Study the drawing (mm; zero at the part's minimum x, y, z) and answer. A direction names the side the tool comes from. Round coordinates to 2 decimals unless told otherwise and drop trailing zeros. Loops run counter-clockwise (first coordinate to the right, second up) from the corner with the lowest first, then second, coordinate; pieces in that order, holes last. Notation, with made-up numbers: (57.5, 70) - (95.5, 70) arc R26 ccw to (95.5, 95) - close; hole circle Ø11 at (12.25, 5.25). An arc over 180 degrees is marked (long way). One line per item, written item: value.
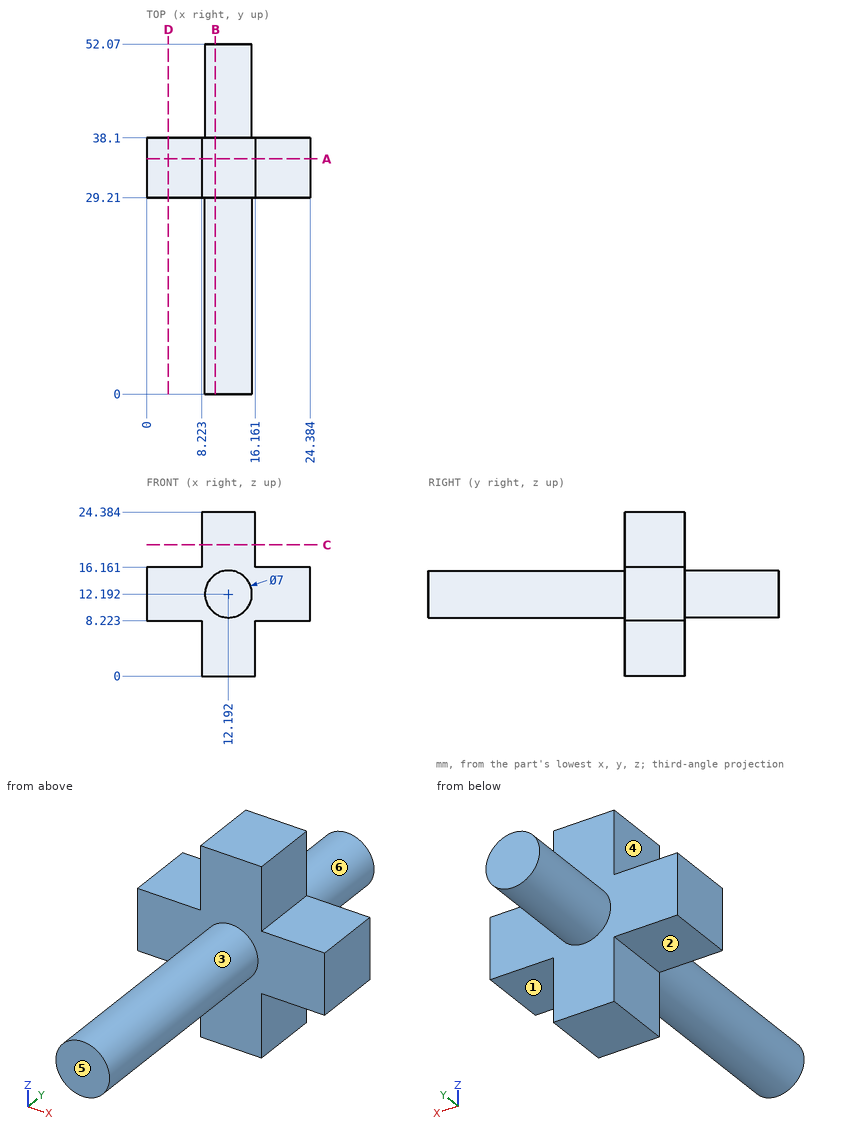
1) A cutting plane is placed at D-D on x = 3.25. Give the vertices of the cut face in (y, z).
Final values:
outline: (29.21, 8.22) - (38.1, 8.22) - (38.1, 16.16) - (29.21, 16.16) - close
2) For a pull along X with two mould halves and no side action, classify the marked faces 4, 5 and 6 as released by +X, released by -X, zero draft, split by the parting line, or undercut.
Final values:
face 4: released by -X
face 5: zero draft
face 6: split by the parting line
3) A cutting plane is placed at B-B on x = 10.25. Give the vertices of the cut face in (y, z).
Final values:
outline: (0, 9.28) - (29.21, 9.28) - (29.21, 0) - (38.1, 0) - (38.1, 9.28) - (52.07, 9.28) - (52.07, 15.1) - (38.1, 15.1) - (38.1, 24.38) - (29.21, 24.38) - (29.21, 15.1) - (0, 15.1) - close
4) For the marked faces 1, 2 and 3, determine the directions among +Z, -Z, +X, -X, +Y, -Y from which every point of the face is accessible in a straight line to the end or side of a thin tool.
Final values:
face 1: -Z, +X, +Y, -Y
face 2: -Z, -X, +Y, -Y
face 3: -Y
5) A cutting plane is placed at C-C on z = 19.5. Give the vertices of the cut face in (x, y).
Final values:
outline: (8.22, 29.21) - (16.16, 29.21) - (16.16, 38.1) - (8.22, 38.1) - close
6) Consider L1, parallel to Y at x = 23, z = 12.5; L2, parallel to Z at x = 3, y = 33; L3, parallel to Z at x = 13, y = 43.5. Determine where each line is inside the solid, lowest interval first.
Final values:
L1: 29.21 to 38.1
L2: 8.22 to 16.16
L3: 8.79 to 15.6
7) Each of these flat-tipped pins is pushed along its axis until it touches: pin 1 Ø2.5 at (x, y) = (22, 35) entering from +Z; pin 2 Ø4 at (y, z) = (35.5, 20) entering from -X; pin 3 Ø10 at (x, z) = (21, 15.5) entering from -Y. Where does it stop, or does it pass through?
Final values:
pin 1: z = 16.16
pin 2: x = 8.22
pin 3: y = 29.21
8) A cutting plane is placed at A-A on y = 35. Give the vertices of the cut face in (x, z), and give its area (3 significant figures).
Final values:
outline: (0, 8.22) - (8.22, 8.22) - (8.22, 0) - (16.16, 0) - (16.16, 8.22) - (24.38, 8.22) - (24.38, 16.16) - (16.16, 16.16) - (16.16, 24.38) - (8.22, 24.38) - (8.22, 16.16) - (0, 16.16) - close
area: 324 mm2
